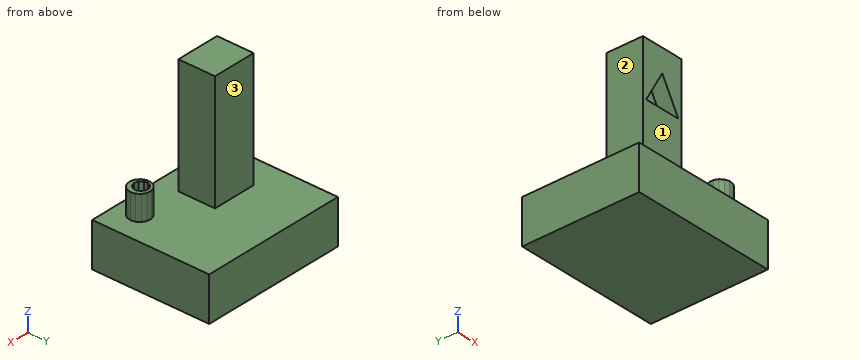
```python
from build123d import *

# Parameters (mm, degrees)
F0_W     = 100
F0_H     = 80
F1_DEPTH = 30
F2_W     = 30
F2_H     = 25
F3_DEPTH = 80
F5_DEPTH = 10
F7_DEPTH = 17
F9_DEPTH = 16


with BuildPart() as f1:
    # F0 (on Top) → F1 (new body)
    with BuildSketch(Plane.XY):
        Rectangle(F0_W, F0_H)
    extrude(amount=F1_DEPTH)

    # F2 (on face) → F3 (join)
    with BuildSketch(Plane.XY.offset(30)):
        with Locations((-15, -12.5)):
            Rectangle(F2_W, F2_H)
    extrude(amount=F3_DEPTH)

    # F4 (on face) → F5 (cut)
    with BuildSketch(Plane.XZ.offset(25)):
        Polygon((-27.5, 72.783122), (-2.5, 72.783122), (-15, 94.433757), align=None)
    extrude(amount=-F5_DEPTH, mode=Mode.SUBTRACT)

    # F6 (on face) → F7 (join)
    with BuildSketch(Plane.XY.offset(30)):
        Polygon((22.943055, -23.5), (22.943055, -26.5), (24.163265, -29.240636), (26.392699, -31.248028), (29.245869, -32.175079), (32.229434, -31.861494), (34.827511, -30.361494), (36.590866, -27.934443), (37.214602, -25), (36.590866, -22.065557), (34.827511, -19.638506), (32.229434, -18.138506), (29.245869, -17.824921), (26.392699, -18.751972), (24.163265, -20.759364), align=None)
    extrude(amount=F7_DEPTH)

    # F8 (on face) → F9 (cut)
    with BuildSketch(Plane.XY.offset(47)):
        Polygon((25.624484, -21.686973), (24.502864, -24.14298), (24.887114, -26.815498), (26.655238, -28.856021), (29.245869, -29.616699), (31.8365, -28.856021), (33.604624, -26.815498), (33.988874, -24.14298), (32.867253, -21.686973), (30.595869, -20.227243), (27.895869, -20.227243), align=None)
    extrude(amount=-F9_DEPTH, mode=Mode.SUBTRACT)


solid = f1.part
```
Check sheet for the modelled part. Datum: model origin and axes. Units: mm. Face numbers are marked on the shaded views. A direction names the side the tool comes from. Coordinates: 2 decimals unless noted, no trailing zeros. Write each loop counter-clockwise with the first axis right and the second up, starting at its lowest first coordinate (ties: lowest second). Pieces come first, ordered by that corner, then holes. Notation, with made-up numbers: M 35,6.25 L 56,6.25 A20 cw 56,12.25 Z; hole C 22.5,31.5 d8. An arc over 180 degrees is marked long. Use one line per item in the form item = value.
Item 1: Sectioned sample at C-C, the plane x = -33. Record the cut outline in (y, z), and give its area (3 significant figures).
Answer below:
outline = M -40,0 L 40,0 L 40,30 L -40,30 Z
area = 2,400 mm^2
Item 2: Gauge pin test, flat ends, axial feed: pin 1 Ø0.9 at (y, z) = (-24.5, 39) entering from -X; pin 2 Ø24 at (x, z) = (-11.5, 86.5) entering from -Y; pin 3 Ø15 at (x, z) = (-9.5, 66.5) entering from +Y. Record the tip position at first contact, or that the pin passes through.
Answer below:
pin_1 = -30
pin_2 = -25
pin_3 = 0
Item 3: Material ranges on L1, parallel to Z at x = 42.5, y = 16.5; L2, parallel to X at y = -9.5, z = 41; L3, parallel to X at y = -20.5, z = 79, recorded low to high. Write a range as from..to.
Answer below:
L1 = 0..30
L2 = -30..0
L3 = -30..-23.91, -6.09..0
Item 4: Sectioned sample at D-D, the plane z = 97. Record the cut outline in (x, y), and give its area (3 significant figures).
Answer below:
outline = M -30,-25 L 0,-25 L 0,0 L -30,0 Z
area = 750 mm^2
Item 5: Sectioned sample at B-B, the plane z = 76.5. Record the cut outline in (x, y), and give its area (3 significant figures).
Answer below:
outline = M -30,-25 L -25.35,-25 L -25.35,-15 L -4.65,-15 L -4.65,-25 L 0,-25 L 0,0 L -30,0 Z
area = 543 mm^2
Item 6: Set-up check for the marked faces 1, 2 and 3: record each of +Z, -Z, +X, -X, +Y, -Y from which the full face is reachable in a straight line by a thin tool's end or side.
Answer below:
face_1 = +Z, -X, -Y
face_2 = +Z, -X, +Y, -Y
face_3 = +Z, +X, -X, +Y
Item 7: Sectioned sample at A-A, the plane y = -4. Record the cut outline in (x, z).
Answer below:
outline = M -50,0 L 50,0 L 50,30 L 0,30 L 0,110 L -30,110 L -30,30 L -50,30 Z
